from build123d import *

# Parameters (mm, degrees)
F0_R           = 30.48
F0_R_2         = 11.049
F1_DEPTH       = 30.48
F2_R           = 15.24
F3_DEPTH       = 15.24
F4_R           = 12.6365
F4_R_2         = 11.049
F5_DEPTH       = 7.112
F6_SIZE2       = 0.254
F6_SIZE        = 0.0680590949
F8_D           = 4.4
F8_CBORE_D     = 8.25
F8_CBORE_DEPTH = 10
F10_D          = 4.0386
F10_DEPTH      = 15.24
F10_TIP        = 1.213317848
F11_R          = 17.4244
F11_R_2        = 14.224
F12_DEPTH      = 1.2954
F13_R          = 0.4064


with BuildPart() as f1:
    # F0 (on Top) → F1 (new body)
    with BuildSketch(Plane.XY):
        Circle(F0_R)
        Circle(F0_R_2, mode=Mode.SUBTRACT)
    extrude(amount=F1_DEPTH)

    # F2 (on face) → F3 (cut)
    with BuildSketch(Plane.XY.offset(30.48)):
        Circle(F2_R)
    extrude(amount=-F3_DEPTH, mode=Mode.SUBTRACT)

    # F4 (on face) → F5 (cut)
    with BuildSketch(Plane(origin=(0, 0, 0), x_dir=(1, 0, 0), z_dir=(0, 0, -1))):
        Circle(F4_R)
        Circle(F4_R_2, mode=Mode.SUBTRACT)
    extrude(amount=-F5_DEPTH, mode=Mode.SUBTRACT)

    # F6
    f6_edges = [f1.edges().sort_by_distance(p)[0] for p in [
        (-11.049, 0, 15.24),
        (-12.6365, 0, 0),
        (-11.049, 0, 7.112),
    ]]
    chamfer(f6_edges, length=F6_SIZE, length2=F6_SIZE2)

    # F8 (through all)
    with Locations(Plane(origin=(0, 0, 0), x_dir=(1, 0, 0), z_dir=(0, 0, -1))):
        with Locations((0, -22), (-22, 0), (0, 22), (22, 0)):
            CounterBoreHole(F8_D / 2, F8_CBORE_D / 2, F8_CBORE_DEPTH)

    # F10
    with Locations(Plane(origin=(0, 0, 0), x_dir=(1, 0, 0), z_dir=(0, 0, -1))):
        with Locations((-19.2474145991, 11.1125), (11.1125, 19.2474145991), (19.2474145991, -11.1125), (-11.1125, -19.2474145991)):
            Hole(F10_D / 2, depth=F10_DEPTH)
            with Locations((0, 0, -(F10_DEPTH + F10_TIP / 2))):  # 118° drill point
                Cone(0, F10_D / 2, F10_TIP, mode=Mode.SUBTRACT)

    # F11 (on face) → F12 (cut)
    with BuildSketch(Plane(origin=(0, 0, 0), x_dir=(1, 0, 0), z_dir=(0, 0, -1))):
        Circle(F11_R)
        Circle(F11_R_2, mode=Mode.SUBTRACT)
    extrude(amount=-F12_DEPTH, mode=Mode.SUBTRACT)

    # F13
    f13_edges = [f1.edges().sort_by_distance(p)[0] for p in [
        (-14.224, 0, 1.2954),
        (-17.4244, 0, 1.2954),
    ]]
    fillet(f13_edges, radius=F13_R)


solid = f1.part
Work out the finished part from the listing and answer in its coordinate system (mm). A direction names the side the tool comes from. Round coordinates to 2 decimals unless told otherwise and drop trailing zeros. Write each loop counter-clockwise with the first axis right and the second up, starting at its lowest first coordinate (ties: lowest second). Pieces come first, ordered by that corner, then holes. Notation, with made-up numbers: (47, -20) -> (65, -20) arc R18 cw to (65, 14) -> close; hole circle Ø8 at (62, 71). An arc over 180 degrees is marked (long way). Write each question's results on one line, items separated by ' | '.
Item 1: A cutting plane is placed at A-A, the plane x = -22.5. Determine the outline of the cut face in (y, z).
Result set:
outline: (-20.56, 0) -> (-4.09, 0) -> (-4.09, 10) -> (-2.14, 10) -> (-2.14, 30.48) -> (-20.56, 30.48) -> close; (2.14, 10) -> (4.09, 10) -> (4.09, 0) -> (20.56, 0) -> (20.56, 30.48) -> (2.14, 30.48) -> close
Item 2: Find the intervals of material crossed by line 1 along X through (y, z) = (-7, 1); line 2 along Y through (x, z) = (18.5, 1.5); line 3 along Y through (x, z) = (0, 18), in increasing order. Write a range as [from, to].
Result set:
line 1: [-29.67, -15.94], [-12.4, -10.52], [10.52, 12.4], [15.94, 29.67] | line 2: [-24.22, -2.18], [2.18, 9.24], [12.99, 24.22] | line 3: [-30.48, -24.2], [-19.8, -15.24], [15.24, 19.8], [24.2, 30.48]
Item 3: Flat-ended cylindrical pins translate along their axes: P1, Ø4, axis at x = 22, z = 6, coming from the -Y side; P2, Ø12.5, axis at x = 3, y = -3, coming from the -Z side; P3, Ø3, axis at x = 8.5, z = 15.5, coming from the +Y side; P4, Ø1.5, axis at x = -8, z = 14, coming from the -Y side. Find the tip coordinate at first contact, or state that the pin passes through.
Result set:
P1: y = -23 | P2: through | P3: y = 29.67 | P4: y = -29.61
Item 4: A cutting plane is placed at C-C, the plane z = 20.5. Determine the outline of the cut face in (x, y).
Result set:
outline: circle Ø60.96 at (0, 0); hole circle Ø4.4 at (-22, 0); hole circle Ø30.48 at (0, 0); hole circle Ø4.4 at (0, -22); hole circle Ø4.4 at (0, 22); hole circle Ø4.4 at (22, 0)
Item 5: Which of the six approach directions +Z, -Z, +X, -X, +Y, -Y give full straight-line access (tool end or side, diameter ignored) to faces 3 (the face through (0.477, 24.148, 20.383)), 4 (the face through (17.88, -0.18, 4.93))?
Result set:
face 3: +Z, -Z | face 4: -Z
Item 6: The mould has two halves that part along X. Classify faces 1 (the face through (13, -13, 0)), 2 (the face through (-10.675, 21.219, 7.727)): +X half, -X half, draft (parallel to the pull), parting line (faces both ways), or undercut.
Result set:
face 1: draft | face 2: undercut
Item 7: A cutting plane is placed at B-B, the plane y = 0. Count the separate pieces of the cut face and the enclosed holes in it, plus the area to 3 significant figures.
Result set:
separate pieces: 4 | enclosed holes: 0 | area: 681 mm^2
